Autodesk Inventor part; units mm, degrees
ref_plane "YZ Plane" through (0, 0, 0) normal (1, 0, 0) x (0, 1, 0)
ref_plane "XZ Plane" through (0, 0, 0) normal (0, 1, 0) x (-1, 0, 0)
ref_plane "XY Plane" through (0, 0, 0) normal (0, 0, 1) x (1, 0, 0)
sketch "Sketch1" plane through (0, 0, 0) normal (0, 0, 1) x (1, 0, 0)
  line L0 (0, 0) -> (0, 101.6)
  line L1 (0, 0) -> (95.25, 0)
  line L2 (95.25, 0) -> (84.2515, 6.35)
  line L3 (95.25, 0) -> (107.95, 0) construction
  line L4 (0, 101.6) -> (12.7, 101.6)
  arc A0 (12.7, 101.6) -> (84.2515, 6.35) centre (110.0717, 100.2457) ccw
  dimension "d0" = 101.6
  dimension "d14" = 12.7
  dimension "d15" = 150
  dimension "d16" = 12.7
  dimension "d28" = 95.25
  dimension "d48" = 97.3812
extrude "Extrusion5" add sketch "Sketch1" along normal blind 152.4
sketch "Sketch5" plane through (0, 0, 0) normal (-1, 0, 0) x (0, 0, 1)
  line L0 (3.81, 97.79) -> (148.59, 97.79)
  line L1 (148.59, 97.79) -> (148.59, 3.175)
  line L2 (148.59, 3.175) -> (3.81, 3.175)
  line L3 (3.81, 3.175) -> (3.81, 97.79)
  line L4 (0, 101.6) -> (152.4, 101.6)
  line L5 (0, 0) -> (0, 101.6)
  line L6 (0, 0) -> (152.4, 0)
  line L7 (152.4, 101.6) -> (152.4, 0)
  dimension "d37" = 3.81
  dimension "d38" = 3.81
  dimension "d39" = 3.175
  dimension "d40" = 3.81
extrude "Extrusion6" cut sketch "Sketch5" against normal blind 101.6 contours L0 L1 L2 L3
fillet "Fillet3" radius 19.05 1 edges at (0, 0, 76.2)
sketch "Sketch6" plane through (0, 97.79, 3.81) normal (0, 0, 1) x (1, 0, 0)
  arc A0 (0, -78.74) -> (19.05, -97.79) centre (19.05, -78.74) ccw
  arc A1 (12.7, 3.81) -> (84.2515, -91.44) centre (77.4018, 0.6973) ccw
  arc A2 (0, -78.74) -> (84.2515, -91.44) centre (63.4925, 56.6564) ccw
  arc A3 (0, -78.74) -> (19.05, -97.79) centre (19.05, -78.74) ccw
  line L0 (95.25, -97.79) -> (19.05, -97.79)
  line L1 (84.2515, -91.44) -> (95.25, -97.79)
  line L2 (19.05, -97.79) -> (95.25, -97.79)
  line L3 (95.25, -97.79) -> (84.2515, -91.44)
  point P0 (0, -97.79)
  dimension "d44" = 149.5443
extrude "Extrusion7" add sketch "Sketch6" along normal up to next
fillet "Fillet4" radius 6.35 12 edges at (41.2021, 6.5727, 148.59) (41.2021, 6.5727, 3.81) (6.3608, 97.79, 148.59) (6.35, 101.6, 152.4) (6.35, 101.6, 0) (6.3608, 97.79, 3.81) (5.5796, 5.5796, 152.4) (0, 60.325, 152.4) (57.15, 0, 152.4) (5.5796, 5.5796, 0) (0, 60.325, 0) (57.15, 0, 0)
sketch "Sketch7" plane through (0, 0, 152.4) normal (0, 0, 1) x (1, 0, 0)
  arc A0 (12.8188, 95.25) -> (84.2515, 6.35) centre (110.0717, 100.2457) ccw
  line L0 (12.7, 101.6) -> (0, 101.6)
  line L1 (12.7, 101.6) -> (72.04, 101.6)
  arc A1 (13.0895, 91.44) -> (70.1837, 11.4086) centre (110.0717, 100.2457) ccw
  arc A2 (12.7, 101.6) -> (24.1017, 54.5046) centre (110.0717, 100.2457) ccw
  line L2 (43.3863, 54.5046) -> (24.1017, 54.5046)
  arc A3 (43.3863, 54.5046) -> (72.04, 101.6) centre (0.6549, 112.7676) ccw
  point P0 (0, 0)
properties part number "Plow"
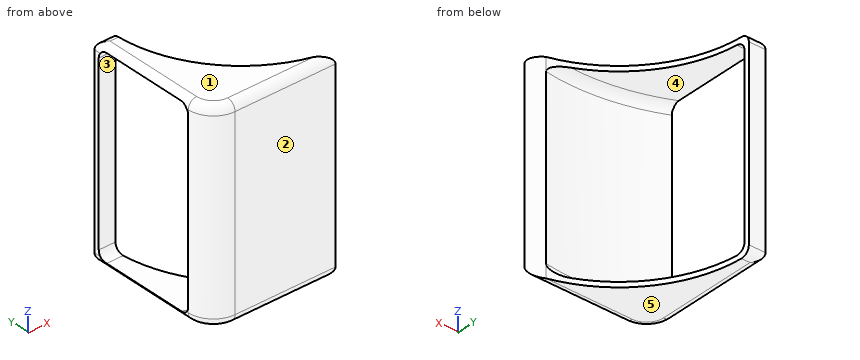
The listing builds one solid part. Answer for the finished solid, in the listing's coordinates (mm). Face numbers are marked on the shaded views. A direction names the side the tool comes from. Coordinates: 2 decimals unless noted, no trailing zeros. Write each loop counter-clockwise with the first axis right and the second up, starting at its lowest first coordinate (ties: lowest second). Pieces come first, ordered by that corner, then holes. Notation, with made-up numbers: (25.5, -20.5) - (71.5, -20.5) arc R29 ccw to (71.5, 15.5) - close; hole circle Ø10 at (18, -38.5). An arc over 180 degrees is marked (long way). Return JSON: item names as keys, results as strings.
1. Which of the six approach directions +Z, -Z, +X, -X, +Y, -Y give full straight-line access (tool end or side, diameter ignored) to the marked faces 4 and 5?
Final values:
{"face 4": "+X", "face 5": "-Z, +X, -X, +Y, -Y"}
2. For a pull along Z with two mould halves and no side action, classify the marked faces 1, 2 and 3 as +Z half, -Z half, draft (parallel to the pull), parting line (faces both ways), or undercut.
Final values:
{"face 1": "+Z half", "face 2": "draft", "face 3": "undercut"}
3. The part is cut by section A-A on z = 54. Determine the outline of the cut face in (x, y).
Final values:
{"outline": "(0, 19.05) arc R19.05 ccw to (19.05, 0) - (95.25, 0) - (84.25, 6.35) arc R149.54 cw to start; (0, 97.79) - (12.72, 97.79) arc R97.38 cw to (12.7, 101.6) - (0, 101.6) - close"}
4. The part is cut by section C-C on x = 86. Determine the outline of the cut face in (y, z).
Final values:
{"outline": "(0, 6.35) arc R6.35 ccw to (5.34, 0.08) - (5.34, 152.32) arc R6.35 ccw to (0, 146.05) - close"}
5. Each of these flat-tipped pins is pushed along its axis until it touches: pin 1 Ø4 at (x, z) = (48.5, 115.5) entering from -Y; pin 2 Ø12 at (x, z) = (64.5, 74.5) entering from +Y; pin 3 Ø14 at (x, z) = (3, 90) entering from -Y; pin 4 Ø1 at (y, z) = (15.5, 33) entering from -X. Where does it stop, or does it pass through?
Final values:
{"pin 1": "y = 0", "pin 2": "y = 5.07", "pin 3": "y = 2.29", "pin 4": "x = 0.25"}
6. The part is cut by section B-B on y = 80. Determine the outline of the cut face in (x, z).
Final values:
{"outline": "(0.53, 3.81) arc R6.35 ccw to (6.35, 0) - (14.82, 0) - (14.82, 3.81) - close; (0.53, 148.59) - (14.82, 148.59) - (14.82, 152.4) - (6.35, 152.4) arc R6.35 ccw to start"}
7. Consider line 1 along Z through (x, y) = (20, 28.5); line 2 along Y through (x, z) = (65, 56); line 3 along Z through (x, y) = (27.5, 14.5). Determine where each line is inside the solid, lowest interval first.
Final values:
{"line 1": "0 to 3.81, 148.59 to 152.4", "line 2": "0 to 4.91", "line 3": "0 to 3.95, 148.45 to 152.4"}
